from build123d import *

# Parameters (mm, degrees)
BOSS_EXTRUDE1_DEPTH = 6.35
SKETCH2_R           = 2.032
CUT_EXTRUDE1_DEPTH  = 166.257012101


with BuildPart() as part:
    # Sketch1 → Boss-Extrude1 (new body)
    with BuildSketch(Plane(origin=(0, 0, 0), x_dir=(1, 0, 0), z_dir=(0, 1, 0))):
        Polygon((90.420598733, 29.997756713), (119.821098733, 29.997756713), (119.821098733, 49.301756713), (128.203098733, 49.301756713), (128.203098733, 29.997756713), (157.603598733, 29.997756713), (157.603598733, -19.151243287), (128.203098733, -19.151243287), (128.203098733, -35.915243287), (119.821098733, -35.915243287), (119.821098733, -19.151243287), (90.420598733, -19.151243287), align=None)
    extrude(amount=BOSS_EXTRUDE1_DEPTH)

    # Sketch2 → Cut-Extrude1 (cut, through all)
    with BuildSketch(Plane(origin=(0, 6.35, 0), x_dir=(1, 0, 0), z_dir=(0, 1, 0))):
        with Locations(Location((124.012098733, -29.311243287, 0), (0, 0, 270))):
            Circle(SKETCH2_R)
        with Locations(Location((124.012098733, 42.697756713, 0), (0, 0, 270))):
            Circle(SKETCH2_R)
    extrude(amount=-CUT_EXTRUDE1_DEPTH, mode=Mode.SUBTRACT)


solid = part.part
Design review of the part built by this model. Coordinates are the model's own, in mm. A direction names the side the tool comes from. Round coordinates to 2 decimals unless told otherwise and drop trailing zeros. Write each loop counter-clockwise with the first axis right and the second up, starting at its lowest first coordinate (ties: lowest second). Pieces come first, ordered by that corner, then holes. Notation, with made-up numbers: (52, -28) -> (106, -28) arc R6 ccw to (106, -20) -> close; hole circle Ø9 at (37.25, 69.5). An arc over 180 degrees is marked (long way). One line per item, written item: value. Start each with the question number.
Q1. The part is to be moulded in two halves that separate along Z. For faces 1 (the face through (105, 3, -29.998)), 2 (the face through (90.421, 3, -5)), 3 (the face through (122.776, 3.219, -44.31)), say which applies: pulls with the +Z half, pulls with the -Z half, needs draft (parallel to the pull), parting line crosses it, or undercut.
Q2. Add section B-B (y = 3.75). Give the boundary of the cut face in (x, z).
Q3. Tool access review of faces 4 (the face through (119.821, 3, -40)), 5 (the face through (143, 3, -29.998)), 6 (the face through (119.821, 3, 28)), 7 (the face through (128.203, 3, 27)): name each direction out of +Z, -Z, +X, -X, +Y, -Y from which nothing blocks a thin tool from reaching the whole face with its end or side.
Q4. Add section C-C (x = 97.5). Give the boundary of the cut face in (y, z), then the cut area to 3 significant figures.
Q5. To check wall thickness, follow probe 1 along Z at (x, y) = (140.5, 2.5); probe 2 along X at (y, z) = (5.25, 28); probe 3 along X at (y, z) = (2.5, 32.5). State the ranges of each line that lie inside material, in increasing order.
Q6. Add section A-A (z = 30). Give the boundary of the cut face in (x, y).
Q7. Insertion check: P1, Ø1.9, axis at y = 4, z = 29.5, coming from the +X side; P2, Ø3, axis at x = 143, y = 5, coming from the -Z side; P3, Ø2.5, axis at x = 124.01, z = 29.31, coming from the -Y side; P4, Ø3, axis at x = 100, y = 4, coming from the +Z side. Each pin has a flat end and moves straight along its axis. Give the tip position at first contact, or say it passes through.
Response:
1. face 1: pulls with the -Z half
1. face 2: needs draft
1. face 3: undercut
2. outline: (90.42, -30) -> (119.82, -30) -> (119.82, -49.3) -> (128.2, -49.3) -> (128.2, -30) -> (157.6, -30) -> (157.6, 19.15) -> (128.2, 19.15) -> (128.2, 35.92) -> (119.82, 35.92) -> (119.82, 19.15) -> (90.42, 19.15) -> close; hole circle Ø4.06 at (124.01, -42.7); hole circle Ø4.06 at (124.01, 29.31)
3. face 4: -Z, -X, +Y, -Y
3. face 5: -Z, +X, +Y, -Y
3. face 6: +Z, -X, +Y, -Y
3. face 7: +Z, +X, +Y, -Y
4. outline: (0, -30) -> (6.35, -30) -> (6.35, 19.15) -> (0, 19.15) -> close
4. area: 312 mm^2
5. probe 1: z = -30 to 19.15
5. probe 2: x = 119.82 to 122.46, 125.56 to 128.2
5. probe 3: x = 119.82 to 128.2
6. outline: (119.82, 0) -> (122.1, 0) -> (122.1, 6.35) -> (119.82, 6.35) -> close; (125.92, 0) -> (128.2, 0) -> (128.2, 6.35) -> (125.92, 6.35) -> close
7. P1: stops at x = 128.2
7. P2: stops at z = -30
7. P3: passes through
7. P4: stops at z = 19.15
